```python
from build123d import *

# Parameters (mm, degrees)
SKETCH1_W                        = 98
SKETCH1_H                        = 60
PCB_BOARD_DEPTH                  = 1.6
SKETCH4_R                        = 1.5
MOUNTING_HOLES_DEPTH             = 1.6
SKETCH5_R                        = 0.5
PCB_HOLES_DEPTH                  = 1.6
SKETCH6_R                        = 0.5
HEADERS_DEPTH                    = 6
SKETCH2_W                        = 97.5
SKETCH2_H                        = 39.7
BLACK_LCD_FRAME_DEPTH            = 9.9
SKETCH7_W                        = 11
SKETCH7_H                        = 3
WHITE_PART_THAT_STICKS_OUT_DEPTH = 2.17
SKETCH3_W                        = 76
SKETCH3_H                        = 26
LCD_SCREEN_DEPTH                 = 0.254
SKETCH8_W                        = 0.692608048
SKETCH8_H                        = 3.684694504
SKETCH8_W_2                      = 0.346304024
SKETCH8_H_2                      = 4.398048289
SKETCH8_W_3                      = 1.171927017
SKETCH8_W_4                      = 1.009844095
SKETCH8_W_5                      = 1.057933222
SKETCH8_W_6                      = 0.585963509
BOSS_EXTRUDE1_DEPTH              = 2.5


with BuildPart() as part:
    # Sketch1 → PCB board (new body)
    with BuildSketch(Plane(origin=(0, 0, 0), x_dir=(1, 0, 0), z_dir=(0, 1, 0))):
        with Locations((-23.16287695, -6.675720991)):
            Rectangle(SKETCH1_W, SKETCH1_H)
    extrude(amount=PCB_BOARD_DEPTH)

    # Sketch4 → Mounting holes (cut)
    with BuildSketch(Plane(origin=(0, 1.6, 0), x_dir=(1, 0, 0), z_dir=(0, 1, 0))):
        with Locations((23.33712305, 20.824279009)):
            Circle(SKETCH4_R)
        with Locations((-69.66287695, -34.175720991)):
            Circle(SKETCH4_R)
        with Locations((-69.66287695, 20.824279009)):
            Circle(SKETCH4_R)
        with Locations((23.33712305, -34.175720991)):
            Circle(SKETCH4_R)
    extrude(amount=-MOUNTING_HOLES_DEPTH, mode=Mode.SUBTRACT)

    # Sketch5 → PCB holes (cut)
    with BuildSketch(Plane(origin=(0, 1.6, 0), x_dir=(1, 0, 0), z_dir=(0, 1, 0))):
        with Locations((15.73712305, -33.575720991)):
            Circle(SKETCH5_R)
        with Locations((13.19712305, -33.575720991)):
            Circle(SKETCH5_R)
        with Locations((10.65712305, -33.575720991)):
            Circle(SKETCH5_R)
        with Locations((8.11712305, -33.575720991)):
            Circle(SKETCH5_R)
        with Locations((5.57712305, -33.575720991)):
            Circle(SKETCH5_R)
        with Locations((3.03712305, -33.575720991)):
            Circle(SKETCH5_R)
        with Locations((0.49712305, -33.575720991)):
            Circle(SKETCH5_R)
        with Locations((-2.04287695, -33.575720991)):
            Circle(SKETCH5_R)
        with Locations((-4.58287695, -33.575720991)):
            Circle(SKETCH5_R)
        with Locations((-7.12287695, -33.575720991)):
            Circle(SKETCH5_R)
        with Locations((-9.66287695, -33.575720991)):
            Circle(SKETCH5_R)
        with Locations((-12.20287695, -33.575720991)):
            Circle(SKETCH5_R)
        with Locations((-14.74287695, -33.575720991)):
            Circle(SKETCH5_R)
        with Locations((-17.28287695, -33.575720991)):
            Circle(SKETCH5_R)
        with Locations((-19.82287695, -33.575720991)):
            Circle(SKETCH5_R)
        with Locations((-22.36287695, -33.575720991)):
            Circle(SKETCH5_R)
    extrude(amount=-PCB_HOLES_DEPTH, mode=Mode.SUBTRACT)

    # Sketch6 → Headers (add)
    with BuildSketch(Plane.XZ):
        with Locations((-22.86287695, 33.575720991)):
            Circle(SKETCH6_R)
        with Locations((-20.32287695, 33.575720991)):
            Circle(SKETCH6_R)
        with Locations((-17.78287695, 33.575720991)):
            Circle(SKETCH6_R)
        with Locations((-15.24287695, 33.575720991)):
            Circle(SKETCH6_R)
        with Locations((-12.70287695, 33.575720991)):
            Circle(SKETCH6_R)
        with Locations((-10.16287695, 33.575720991)):
            Circle(SKETCH6_R)
        with Locations((-7.62287695, 33.575720991)):
            Circle(SKETCH6_R)
        with Locations((-5.08287695, 33.575720991)):
            Circle(SKETCH6_R)
        with Locations((-2.54287695, 33.575720991)):
            Circle(SKETCH6_R)
        with Locations((-0.00287695, 33.575720991)):
            Circle(SKETCH6_R)
        with Locations((2.53712305, 33.575720991)):
            Circle(SKETCH6_R)
        with Locations((5.07712305, 33.575720991)):
            Circle(SKETCH6_R)
        with Locations((7.61712305, 33.575720991)):
            Circle(SKETCH6_R)
        with Locations((10.15712305, 33.575720991)):
            Circle(SKETCH6_R)
        with Locations((12.69712305, 33.575720991)):
            Circle(SKETCH6_R)
        with Locations((15.23712305, 33.575720991)):
            Circle(SKETCH6_R)
    extrude(amount=HEADERS_DEPTH)

    # Sketch2 → Black LCD frame (add)
    with BuildSketch(Plane(origin=(0, 1.6, 0), x_dir=(1, 0, 0), z_dir=(0, 1, 0))):
        with Locations((-23.16287695, -6.675720991)):
            Rectangle(SKETCH2_W, SKETCH2_H)
    extrude(amount=BLACK_LCD_FRAME_DEPTH)

    # Sketch7 → White part that sticks out (add)
    with BuildSketch(Plane.ZY.offset(71.91287695)):
        with Locations((5.5, 3.1)):
            Rectangle(SKETCH7_W, SKETCH7_H)
    extrude(amount=WHITE_PART_THAT_STICKS_OUT_DEPTH)

    # Sketch3 → LCD screen (cut)
    with BuildSketch(Plane(origin=(0, 11.5, 0), x_dir=(1, 0, 0), z_dir=(0, 1, 0))):
        with Locations((-23.766549937, -6.888251248)):
            Rectangle(SKETCH3_W, SKETCH3_H)
    extrude(amount=-LCD_SCREEN_DEPTH, mode=Mode.SUBTRACT)

    # Sketch8 → Boss-Extrude1 (add)
    with BuildSketch(Plane.XZ):
        with Locations((-65.871568973, 28.956578117)):
            Rectangle(SKETCH8_W, SKETCH8_H)
        with Locations((-65.698416961, -15.916426138)):
            Rectangle(SKETCH8_W_2, SKETCH8_H_2)
        with Locations((-26.349706369, -15.916426138)):
            Rectangle(SKETCH8_W_3, SKETCH8_H_2)
        with Locations((17.054029789, -15.916426138)):
            Rectangle(SKETCH8_W_4, SKETCH8_H_2)
        with Locations((18.087918447, 28.956578117)):
            Rectangle(SKETCH8_W_5, SKETCH8_H)
        with Locations((-26.642688123, 28.956578117)):
            Rectangle(SKETCH8_W_6, SKETCH8_H)
    extrude(amount=BOSS_EXTRUDE1_DEPTH)


solid = part.part
```
Input: part model. Units: mm. Frame: model coordinates. A direction names the side the tool comes from. Round coordinates to 2 decimals unless told otherwise and drop trailing zeros. Write each loop counter-clockwise with the first axis right and the second up, starting at its lowest first coordinate (ties: lowest second). Pieces come first, ordered by that corner, then holes. Notation, with made-up numbers: (36.25, 86) - (75.25, 86) arc R14 ccw to (75.25, 99) - close; hole circle Ø11 at (42, 54). An arc over 180 degrees is marked (long way). Write item = value, one per line.
(1) Contact query for flat-ended pins moving along their axis: pin 1 Ø2 at (y, z) = (1, 14.5) entering from -X; pin 2 Ø0.8 at (y, z) = (-2, -15.5) entering from +X; pin 3 Ø0.8 at (y, z) = (-1.5, -15) entering from -X; pin 4 Ø2.5 at (x, z) = (-69.66, -20.82) entering from +Y. Output: stop coordinate, or through.
Geometry check:
pin_1 = -72.16
pin_2 = 17.56
pin_3 = -65.87
pin_4 = through
(2) Section query A-A on z = 22. Output: boundary loops of the cut face in (x, y), then the cut area to 3 significant figures.
Geometry check:
outline = (-72.16, 0) - (25.84, 0) - (25.84, 1.6) - (25.59, 1.6) - (25.59, 11.5) - (-71.91, 11.5) - (-71.91, 1.6) - (-72.16, 1.6) - close
area = 1,120 mm^2
(3) Section query B-B on x = -64.5. Output: boundary loops of the cut face in (y, z), then the cut area to 3 significant figures.
Geometry check:
outline = (0, -23.32) - (1.6, -23.32) - (1.6, -13.17) - (11.5, -13.17) - (11.5, 26.53) - (1.6, 26.53) - (1.6, 36.68) - (0, 36.68) - close
area = 489 mm^2
(4) Section query D-D on y = 8. Output: boundary loops of the cut face in (x, z).
Geometry check:
outline = (-71.91, -13.17) - (25.59, -13.17) - (25.59, 26.53) - (-71.91, 26.53) - close
(5) Material intervals for probe 1 along Z at (x, y) = (-70, 1.25); probe 2 along X at (y, z) = (1, 34.5); probe 3 along Y at (x, z) = (-11, 31), sorted ascending.
Geometry check:
probe_1 = -23.32 to -22.29, -19.36 to 32.71, 35.64 to 36.68
probe_2 = -72.16 to -71.13, -68.2 to 21.87, 24.8 to 25.84
probe_3 = 0 to 1.6
(6) Pull-direction query (Z, two-part tool) for faces 1 (the cylindrical face through (23.01, 0.81, 35.64)), 2 (the flat face through (-26.936, -1, 29)), 3 (the cylindrical face through (21.84, 0.81, -20.89)), 4 (the flat face through (-73, 3, 11)); classes: +Z half, -Z half, draft (parallel to the pull), parting line (faces both ways), or undercut.
Geometry check:
face_1 = undercut
face_2 = draft
face_3 = undercut
face_4 = +Z half
(7) Access query for faces 5 (the flat face through (-24, 6, 26.526)), 6 (the flat face through (17.559, -1, 29)), 7 (the flat face through (-24, 6, -13.174)). Directions: +Z, -Z, +X, -X, +Y, -Y. A direction counts if a zero-diameter tool reaches every point of the face in a straight line with its end or side. Return the directions, or none.
Geometry check:
face_5 = +Z, +X, -X, +Y
face_6 = +Z, -Y
face_7 = -Z, +X, -X, +Y
(8) Section query C-C on y = -3.5. State how many separate pieces and enclosed holes the cut face has, then the cut area to 3 significant figures.
Geometry check:
separate_pieces = 16
enclosed_holes = 0
area = 12.6 mm^2
